```python
from build123d import *

# Parameters (mm, degrees)
SKETCH1_R           = 25
SKETCH1_R_2         = 1.25
SKETCH1_R_3         = 3
BOSS_EXTRUDE1_DEPTH = 3


with BuildPart() as part:
    # Sketch1 → Boss-Extrude1 (new body)
    with BuildSketch(Plane.XY):
        Circle(SKETCH1_R)
        with Locations((0, 22.5)):
            Circle(SKETCH1_R_2, mode=Mode.SUBTRACT)
        Circle(SKETCH1_R_3, mode=Mode.SUBTRACT)
        with Locations((22.5, 0)):
            Circle(SKETCH1_R_2, mode=Mode.SUBTRACT)
        with Locations((0, -22.5)):
            Circle(SKETCH1_R_2, mode=Mode.SUBTRACT)
        with Locations((-22.5, 0)):
            Circle(SKETCH1_R_2, mode=Mode.SUBTRACT)
        with BuildLine():
            Line((4.39039635, 17.512781765), (3.066480056, 12.042499157))
            ThreePointArc((3.066480056, 12.042499157), (3.243806018, 10.234010462), (4.506349736, 8.927083066))
            ThreePointArc((4.506349736, 8.927083066), (7.071067812, 7.071067812), (8.927083066, 4.506349736))
            ThreePointArc((8.927083066, 4.506349736), (10.234010462, 3.243806018), (12.042499157, 3.066480056))
            Line((12.042499157, 3.066480056), (17.512781765, 4.39039635))
            ThreePointArc((17.512781765, 4.39039635), (18.69880908, 5.306187253), (18.808282105, 6.800626756))
            ThreePointArc((18.808282105, 6.800626756), (14.142135624, 14.142135624), (6.800626756, 18.808282105))
            ThreePointArc((6.800626756, 18.808282105), (5.306187253, 18.69880908), (4.39039635, 17.512781765))
        make_face(mode=Mode.SUBTRACT)
        with BuildLine():
            Line((4.39039635, -17.512781765), (3.066480056, -12.042499157))
            ThreePointArc((3.066480056, -12.042499157), (3.243806018, -10.234010462), (4.506349736, -8.927083066))
            ThreePointArc((4.506349736, -8.927083066), (7.071067812, -7.071067812), (8.927083066, -4.506349736))
            ThreePointArc((8.927083066, -4.506349736), (10.234010462, -3.243806018), (12.042499157, -3.066480056))
            Line((12.042499157, -3.066480056), (17.512781765, -4.39039635))
            ThreePointArc((17.512781765, -4.39039635), (18.69880908, -5.306187253), (18.808282105, -6.800626756))
            ThreePointArc((18.808282105, -6.800626756), (14.142135624, -14.142135624), (6.800626756, -18.808282105))
            ThreePointArc((6.800626756, -18.808282105), (5.306187253, -18.69880908), (4.39039635, -17.512781765))
        make_face(mode=Mode.SUBTRACT)
        with BuildLine():
            Line((-17.512781765, -4.39039635), (-12.042499157, -3.066480056))
            ThreePointArc((-12.042499157, -3.066480056), (-10.234010462, -3.243806018), (-8.927083066, -4.506349736))
            ThreePointArc((-8.927083066, -4.506349736), (-7.071067812, -7.071067812), (-4.506349736, -8.927083066))
            ThreePointArc((-4.506349736, -8.927083066), (-3.243806018, -10.234010462), (-3.066480056, -12.042499157))
            Line((-3.066480056, -12.042499157), (-4.39039635, -17.512781765))
            ThreePointArc((-4.39039635, -17.512781765), (-5.306187253, -18.69880908), (-6.800626756, -18.808282105))
            ThreePointArc((-6.800626756, -18.808282105), (-14.142135624, -14.142135624), (-18.808282105, -6.800626756))
            ThreePointArc((-18.808282105, -6.800626756), (-18.69880908, -5.306187253), (-17.512781765, -4.39039635))
        make_face(mode=Mode.SUBTRACT)
        with BuildLine():
            Line((-4.39039635, 17.512781765), (-3.066480056, 12.042499157))
            ThreePointArc((-3.066480056, 12.042499157), (-3.243806018, 10.234010462), (-4.506349736, 8.927083066))
            ThreePointArc((-4.506349736, 8.927083066), (-7.071067812, 7.071067812), (-8.927083066, 4.506349736))
            ThreePointArc((-8.927083066, 4.506349736), (-10.234010462, 3.243806018), (-12.042499157, 3.066480056))
            Line((-12.042499157, 3.066480056), (-17.512781765, 4.39039635))
            ThreePointArc((-17.512781765, 4.39039635), (-18.69880908, 5.306187253), (-18.808282105, 6.800626756))
            ThreePointArc((-18.808282105, 6.800626756), (-14.142135624, 14.142135624), (-6.800626756, 18.808282105))
            ThreePointArc((-6.800626756, 18.808282105), (-5.306187253, 18.69880908), (-4.39039635, 17.512781765))
        make_face(mode=Mode.SUBTRACT)
    extrude(amount=BOSS_EXTRUDE1_DEPTH)


solid = part.part
```
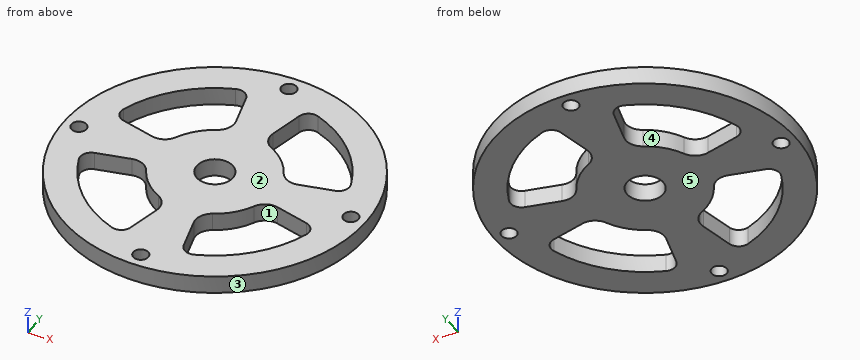
Geometry: final body of the model. Coordinates: model frame, mm. Face numbers are marked on the shaded views. A direction names the side the tool comes from. Coordinates: 2 decimals unless noted, no trailing zeros. Order: outer loops, then holes, each group sorted by start corner. A loop starts at its lowest first (then second) coordinate and runs counter-clockwise, first axis right, second up. Notation, with made-up numbers: (88.5, 59) -> (137.5, 59) arc R7 cw to (137.5, 63) -> close; hole circle Ø6 at (10.25, -13). An arc over 180 degrees is marked (long way). Use CSV: the item, a comma, the result in double quotes.
1) Section A-A on y = -10. Output: boundary loops of the cut face in (x, z), then the cut area to 3 significant figures.
Findings:
outline,"(-22.91, 0) -> (-17.32, 0) -> (-17.32, 3) -> (-22.91, 3) -> close; (-3.37, 0) -> (3.37, 0) -> (3.37, 3) -> (-3.37, 3) -> close; (17.32, 0) -> (22.91, 0) -> (22.91, 3) -> (17.32, 3) -> close"
area,"53.7 mm^2"
2) Pin query (flat end, axial travel): pin 1 Ø2 at (x, y) = (0, 22.5) entering from +Z; pin 2 Ø1 at (y, z) = (4, 1.5) entering from -X. Return the tip coordinate at first contact, or that it passes through.
Findings:
pin 1,"passes through"
pin 2,"stops at x = -24.75"
3) Access query for the marked faces 1 and 2. Directions: +Z, -Z, +X, -X, +Y, -Y. A direction counts if a zero-diameter tool reaches every point of the face in a straight line with its end or side. Return the directions, or none.
Findings:
face 1,"+Z, -Z"
face 2,"+Z, +X, -X, +Y, -Y"
4) Section C-C on y = 0. Output: boundary loops of the cut face in (x, z), then the cut area to 3 significant figures.
Findings:
outline,"(-25, 0) -> (-23.75, 0) -> (-23.75, 3) -> (-25, 3) -> close; (-21.25, 0) -> (-3, 0) -> (-3, 3) -> (-21.25, 3) -> close; (3, 0) -> (21.25, 0) -> (21.25, 3) -> (3, 3) -> close; (23.75, 0) -> (25, 0) -> (25, 3) -> (23.75, 3) -> close"
area,"117 mm^2"
5) Line query: line 1 (X direction, y = 17.5, z = 0.2); line 2 (X direction, y = 1, z = 1.7); line 3 (X direction, y = -18, z = 1.85). Output: solid intervals per line, ascending.
Findings:
line 1,"x = -17.85 to -9.68, -4.39 to 4.39, 9.68 to 17.85"
line 2,"x = -24.98 to -23.25, -21.75 to -2.83, 2.83 to 21.75, 23.25 to 24.98"
line 3,"x = -17.35 to -8.72, -4.59 to 4.59, 8.72 to 17.35"
6) Section B-B on x = -22. Output: boundary loops of the cut face in (y, z), then the cut area to 3 significant figures.
Findings:
outline,"(-11.87, 0) -> (-1.15, 0) -> (-1.15, 3) -> (-11.87, 3) -> close; (1.15, 0) -> (11.87, 0) -> (11.87, 3) -> (1.15, 3) -> close"
area,"64.4 mm^2"
7) Section D-D on y = -22.5. Output: boundary loops of the cut face in (x, z).
Findings:
outline,"(-10.9, 0) -> (-1.25, 0) -> (-1.25, 3) -> (-10.9, 3) -> close; (1.25, 0) -> (10.9, 0) -> (10.9, 3) -> (1.25, 3) -> close"
8) Mould query, pull axis Y, two halves, no side actions, for the marked faces 3, 4 and 5. Classes: +Y half, -Y half, draft (parallel to the pull), parting line (faces both ways), or undercut.
Findings:
face 3,"parting line"
face 4,"undercut"
face 5,"draft"
